Geometry: final body of the model. Coordinates: model frame, mm. Face numbers are marked on the shaded views. A direction names the side the tool comes from. Round coordinates to 2 decimals unless told otherwise and drop trailing zeros. Loops run counter-clockwise (first coordinate to the right, second up) from the corner with the lowest first, then second, coordinate; pieces in that order, holes last. Notation, with made-up numbers: M -15.5,46 L -9.5,46 A13 ccw -9.5,70 Z; hole C 2,24 d2. An arc over 180 degrees is marked long. Answer as a JSON object with one key per item and string values.
Autodesk Fusion 360 part; units mm, degrees
sketch "草图1" plane through (0, 0, 0) normal (1, 0, 0) x (0, 1, 0)
  circle A0 centre (0, 36) radius 4.5
  line L0 (-20, 0) -> (-30, 0)
  line L1 (-30, 0) -> (-46.5, 0)
  line L2 (-46.5, 0) -> (-46.5, 8)
  line L3 (-46.5, 8) -> (-28.9137, 8)
  line L4 (30, 0) -> (46.5, 0)
  line L5 (46.5, 0) -> (46.5, 8)
  line L6 (46.5, 8) -> (28.9137, 8)
  line L7 (30, 0) -> (20, 0)
  arc A1 (30, 0) -> (-30, 0) centre (0, 0) ccw
  arc A2 (20, 0) -> (-20, 0) centre (0, 0) ccw
  line L8 (0, 110) -> (0, -20) construction
  line L9 (-9, 36) -> (-9, 28.6182)
  line L10 (9, 36) -> (9, 28.6182)
  arc A3 (9, 36) -> (-9, 36) centre (0, 36) ccw
  dimension "d1" = 93
  dimension "d2" = 20
  dimension "d3" = 30
  dimension "d4" = 8
  dimension "d5" = 8
  dimension "d6" = 36
  dimension "d7" = 18
  dimension "d8" = 9
extrude "拉伸1" add sketch "草图1" along normal mid plane 18 contours L1 L2 L3 A1 | L4 L5 L6 A1 makes body 1 at (-3, 40.6379, 8) makes body 2 at (-3, -40.6379, 8)
extrude "拉伸2" add sketch "草图1" along normal mid plane 60 contours L0 L7 A1 A2 bodies 1 2
extrude "拉伸3" add sketch "草图1" along normal blind 8 separate body contours A1 L9 L10 A3 makes body 3
move_body "移动1" bodies 3 to x (1, 0, 0) y (0, 1, 0) z (0, 0, 1) at (22, 0, 0)
copy_body "复制和粘贴实体1" bodies 3 makes body 4
move_body "移动2" bodies 4 to x (1, 0, 0) y (0, 1, 0) z (0, 0, 1) at (-52, 0, 0)
fillet "圆角1" radius 9 4 edges at (9, -46.5, 4) (-9, -46.5, 4) (9, 46.5, 4) (-9, 46.5, 4) on bodies 1
sketch "草图2" plane through (0, 0, 8) normal (0, 0, 1) x (-1, 0, 0)
  arc A0 (-9, -37.5) -> (9, -37.5) centre (0, -37.5) ccw
  line L0 (9, -37.5) -> (9, -28.9137)
  line L1 (9, -28.9137) -> (-9, -28.9137)
  line L2 (-9, -28.9137) -> (-9, -37.5)
  circle A1 centre (0, -37.5) radius 4.5
  circle A2 centre (0, 37.5) radius 4.5
  line L3 (55, 0) -> (-41.8167, 0) construction
  dimension "d17" = 9
  dimension "d18" = 75
extrude "拉伸4" cut sketch "草图2" against normal through all contours A1 | A2 bodies 1
combine "合并1" operation add target body 1 tool bodies 4 3
equation "d1 = 75 mm + 18 mm"
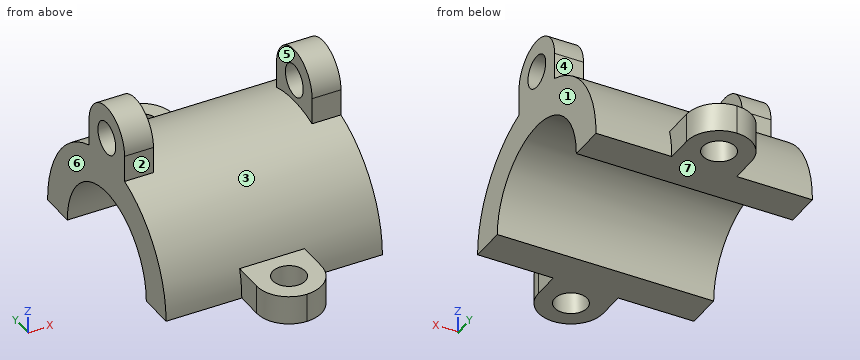
1) Reachability of the marked faces 1, 2, 3 and 4 from +Z, -Z, +X, -X, +Y, -Y: full face, straight path, thin tool, end or side. Return the list, or none.
Results:
{"face 1": "+Z, -Z, +X, +Y, -Y", "face 2": "+Z, +X, -X, -Y", "face 3": "+Z", "face 4": "+Z, +X, -X, +Y"}
2) Ray query, line 1 (Z direction, x = 25.75, y = 0); line 2 (Y direction, x = 0, z = 2.5); line 3 (Y direction, x = 0, z = 5). Return the intervals inside material, ascending.
Results:
{"line 1": "20 to 31.5, 40.5 to 45", "line 2": "-46.5 to -42, -33 to -19.84, 19.84 to 33, 42 to 46.5", "line 3": "-46.5 to -42, -33 to -19.36, 19.36 to 33, 42 to 46.5"}
3) Section query A-A (y = 0). Return the cut outline in (x, z).
Results:
{"outline": "M -30,20 L 30,20 L 30,31.5 L 22,31.5 L 22,30 L -22,30 L -22,31.5 L -30,31.5 Z; M -30,40.5 L -22,40.5 L -22,45 L -30,45 Z; M 22,40.5 L 30,40.5 L 30,45 L 22,45 Z"}
4) Pin query (flat end, axial travel): P1, Ø9, axis at x = -3.5, y = 36.5, coming from the +Z side; P2, Ø3.5, axis at x = -27, z = 30.5, coming from the +Y side; P3, Ø4, axis at y = -35, z = 4.5, coming from the +X side; P4, Ø7, axis at x = 0, y = 37.5, coming from the +Z side. Return the tip coordinate at first contact, or that it passes through.
Results:
{"P1": "z = 8", "P2": "y = 9", "P3": "x = 9", "P4": "through"}
5) Section query B-B (z = 6). Count the separate pieces of the cut face and the enclosed holes in it, and give its area (3 significant figures).
Results:
{"separate pieces": "2", "enclosed holes": "2", "area": "1,660 mm2"}
6) Pull-direction query (X, two-part tool) for the marked faces 5, 6 and 7; classes: +X half, -X half, draft (parallel to the pull), parting line (faces both ways), or undercut.
Results:
{"face 5": "undercut", "face 6": "-X half", "face 7": "draft"}
7) Section query D-D (z = 42.5). Return the cut outline in (x, y).
Results:
{"outline": "M -30,-6.22 L -22,-6.22 L -22,6.22 L -30,6.22 Z; M 22,-6.22 L 30,-6.22 L 30,6.22 L 22,6.22 Z"}
8) Section query C-C (x = 25). Return the cut outline in (y, z).
Results:
{"outline": "M -30,0 L -20,0 A20 cw 20,0 L 30,0 A30 ccw 9,28.62 L 9,36 A9 ccw -9,36 L -9,28.62 A30 ccw Z; hole C 0,36 d9"}
